Part print with two shaded views. Sizes in mm from the minimum x, y, z corner. Round coordinates to 2 decimals unless told otherwise and drop trailing zeros. Loops run counter-clockwise (first coordinate to the right, second up) from the corner with the lowest first, then second, coordinate; pieces in that order, holes last. Notation, with made-up numbers: (63, 0) -> (110, 0) arc R9 ccw to (110, 4) -> close; hole circle Ø5 at (27, -9). An arc over 180 degrees is marked (long way). Answer as a JSON object with one key per item and string values. Group by question number.
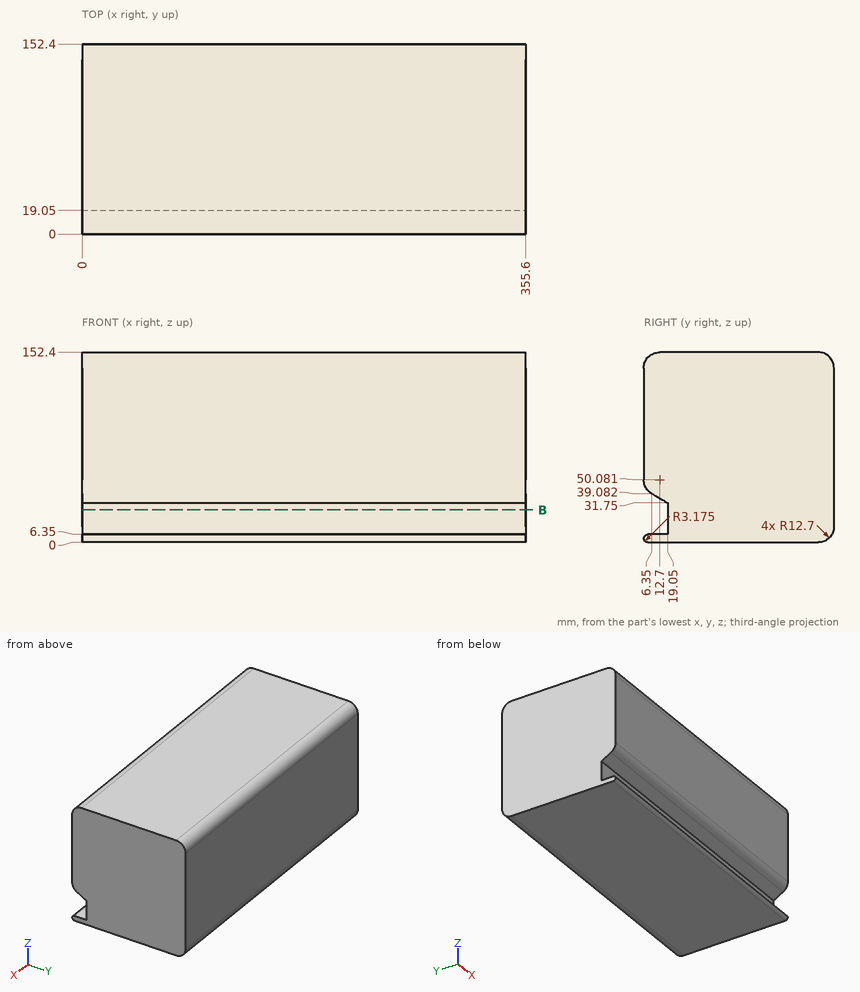
Item 1: Drill centre lines: line 1 (Y direction, x = 325.5, z = 25.5); line 2 (Y direction, x = 168, z = 140). Where is each one in solid material? Low to high.
Item 2: Band-saw the part on B-B, the plane z = 26. List the corners of the cut face in (x, y).
Item 3: Drop flat-ended pins along their axis: pin 1 Ø1 at (x, z) = (291, 48.5) entering from -Y; pin 2 Ø12.5 at (x, z) = (221.5, 15) entering from -Y. Give the stop position or say it passes through.
Entries:
{
 "1": {"line 1": "19.05 to 152.4", "line 2": "0 to 152.4"},
 "2": {"outline": "(0, 19.05) -> (355.6, 19.05) -> (355.6, 152.4) -> (0, 152.4) -> close"},
 "3": {"pin 1": "y = 0.05", "pin 2": "y = 19.05"}
}
